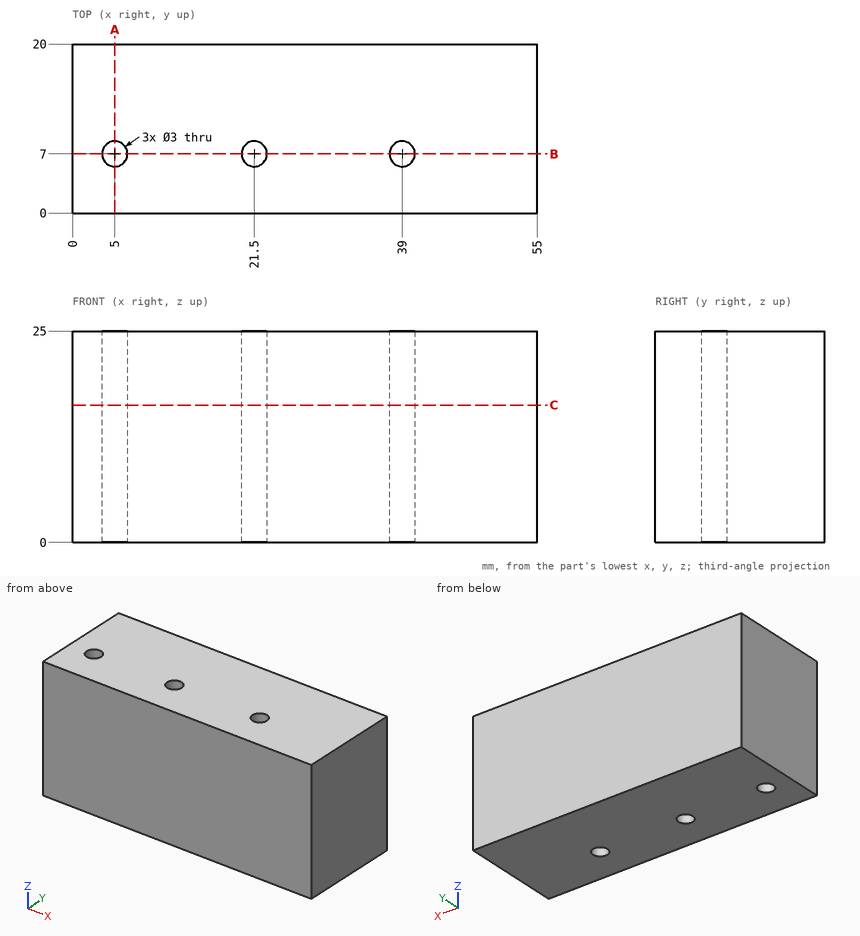
Input: dimensioned drawing with shaded views. Units: mm. Origin: part minimum x, y, z. Give positions to 0.01 mm unless a question says otherwise; leave off trailing zeros. Write each loop counter-clockwise with the first axis right and the second up, starting at its lowest first coordinate (ties: lowest second). Pieces come first, ordered by that corner, then holes. Notation, with made-up numbers: (38, -30.5) - (56, -30.5) arc R8 cw to (56, -25.5) - close; hole circle Ø1 at (66.25, 24.25). An arc over 180 degrees is marked (long way). One line per item, written item: value. Start each with the question number.
Q1. Section query A-A, the plane x = 5. Return the cut outline in (y, z), then the cut area to 3 significant figures.
Q2. Section query C-C, the plane z = 16.25. Return the cut outline in (x, y).
Q3. Material intervals for probe 1 along Y at (x, z) = (5, 11.25); probe 2 along X at (y, z) = (5.75, 1.5); probe 3 along Y at (x, z) = (39.5, 22.75), sorted ascending. Write a range as from..to.
Q4. Section query B-B, the plane y = 7. Return the cut outline in (x, z).
Answer:
1. outline: (0, 0) - (5.5, 0) - (5.5, 25) - (0, 25) - close; (8.5, 0) - (20, 0) - (20, 25) - (8.5, 25) - close
1. area: 425 mm2
2. outline: (0, 0) - (55, 0) - (55, 20) - (0, 20) - close; hole circle Ø3 at (5, 7); hole circle Ø3 at (21.5, 7); hole circle Ø3 at (39, 7)
3. probe 1: y = 0..5.5, 8.5..20
3. probe 2: x = 0..4.17, 5.83..20.67, 22.33..38.17, 39.83..55
3. probe 3: y = 0..5.59, 8.41..20
4. outline: (0, 0) - (3.5, 0) - (3.5, 25) - (0, 25) - close; (6.5, 0) - (20, 0) - (20, 25) - (6.5, 25) - close; (23, 0) - (37.5, 0) - (37.5, 25) - (23, 25) - close; (40.5, 0) - (55, 0) - (55, 25) - (40.5, 25) - close
